from build123d import *

# Parameters (mm, degrees)
SKETCH3_R           = 4.7625
CUT_EXTRUDE1_DEPTH  = 25.4
SKETCH4_W           = 15.24
SKETCH4_H           = 15.24
BOSS_EXTRUDE1_DEPTH = 12.7


with BuildPart() as part:
    # Sketch1 → Revolve2 (revolve)
    with BuildSketch(Plane.XY, mode=Mode.PRIVATE) as revolve2_sk:
        Polygon((0, 0), (152.4, 0), (152.4, 12.7), (0, 15.875), align=None)
    revolve(revolve2_sk.sketch.rotate(Axis((0, 0, 0), (1, 0, 0)), 90), axis=Axis((0, 0, 0), (1, 0, 0)))

    # Sketch3 → Cut-Extrude1 (cut)
    with BuildSketch(Plane(origin=(152.4, 0, 0), x_dir=(0, 0, -1), z_dir=(1, 0, 0))):
        Circle(SKETCH3_R)
    extrude(amount=-CUT_EXTRUDE1_DEPTH, mode=Mode.SUBTRACT)

    # Sketch4 → Boss-Extrude1 (add)
    with BuildSketch(Plane.ZY):
        Rectangle(SKETCH4_W, SKETCH4_H)
    extrude(amount=BOSS_EXTRUDE1_DEPTH)


solid = part.part
Read the model definition and answer for the solid it produces. Units are mm, in the model's axes. A direction names the side the tool comes from. Round coordinates to 2 decimals unless told otherwise and drop trailing zeros. Order: outer loops, then holes, each group sorted by start corner. A loop starts at its lowest first (then second) coordinate and runs counter-clockwise, first axis right, second up.
1) For faces 1 (the face through (-6, 7.62, 0)), 2 (the face through (-6, 0, -7.62)), 3 (the face through (-6, 0, 7.62)), 4 (the face through (75.133, -0.629, -14.296)), 5 (the face through (-12.7, 0, 0)), determine the directions among +Z, -Z, +X, -X, +Y, -Y from which every point of the face is accessible in a straight line to the end or side of a thin tool.
2) The part is cut by section A-A on z = 0. Write down the section's boundary in (x, y) (1 decimal).
3) The part is cut by section C-C on x = 14.5. Write down the section's boundary in (y, z).
4) The mould has two halves that part along Y. Classify faces 6 (the face through (139.88, -2.9, 3.78)), 7 (the face through (127, 0, 0)), 8 (the face through (-6, -7.62, 0)), 9 (the face through (152.4, 0, -5)): released by +Y, released by -Y, zero draft, split by the parting line, or undercut.
5) Straight lines are drawn through the part: L1, parallel to X at y = -11, z = -1; L2, parallel to Y at x = 136.75, z = 0; L3, parallel to Y at x = 145, z = 0. For each, find the intervals that lie inside material, in ascending order.
6) The part is cut by section D-D on x = 130. Write down the section's boundary in (y, z) (1 decimal), plus the area to 3 significant figures.
7) Flat-ended cylindrical pins translate along their axes: pin 1 (2 mm diameter, centred on x = 56.5, z = 3.5, fed in from -Y) (3 decimals); pin 2 (8 mm diameter, centred on x = 87.5, y = 6.5, fed in from -Z); pin 3 (4 mm diameter, centred on x = 19.5, z = -7, fed in from -Y). Find the tip coordinate at first contact, or state that the pin passes through.
Resolved:
1. face 1: +Z, -Z, -X, +Y
1. face 2: -Z, -X, +Y, -Y
1. face 3: +Z, -X, +Y, -Y
1. face 4: +X
1. face 5: +Z, -Z, -X, +Y, -Y
2. outline: (-12.7, -7.6) - (0, -7.6) - (0, -15.9) - (152.4, -12.7) - (152.4, -4.8) - (127, -4.8) - (127, 4.8) - (152.4, 4.8) - (152.4, 12.7) - (0, 15.9) - (0, 7.6) - (-12.7, 7.6) - close
3. outline: circle Ø31.15 at (0, 0)
4. face 6: undercut
4. face 7: undercut
4. face 8: released by -Y
4. face 9: zero draft
5. L1: x = 0 to 152.4
5. L2: y = -13.03 to -4.76, 4.76 to 13.03
5. L3: y = -12.85 to -4.76, 4.76 to 12.85
6. outline: circle Ø26.3 at (0, 0); hole circle Ø9.5 at (0, 0)
6. area: 473 mm2
7. pin 1: stops at y = -14.485
7. pin 2: stops at z = -13.83
7. pin 3: stops at y = -14.64
